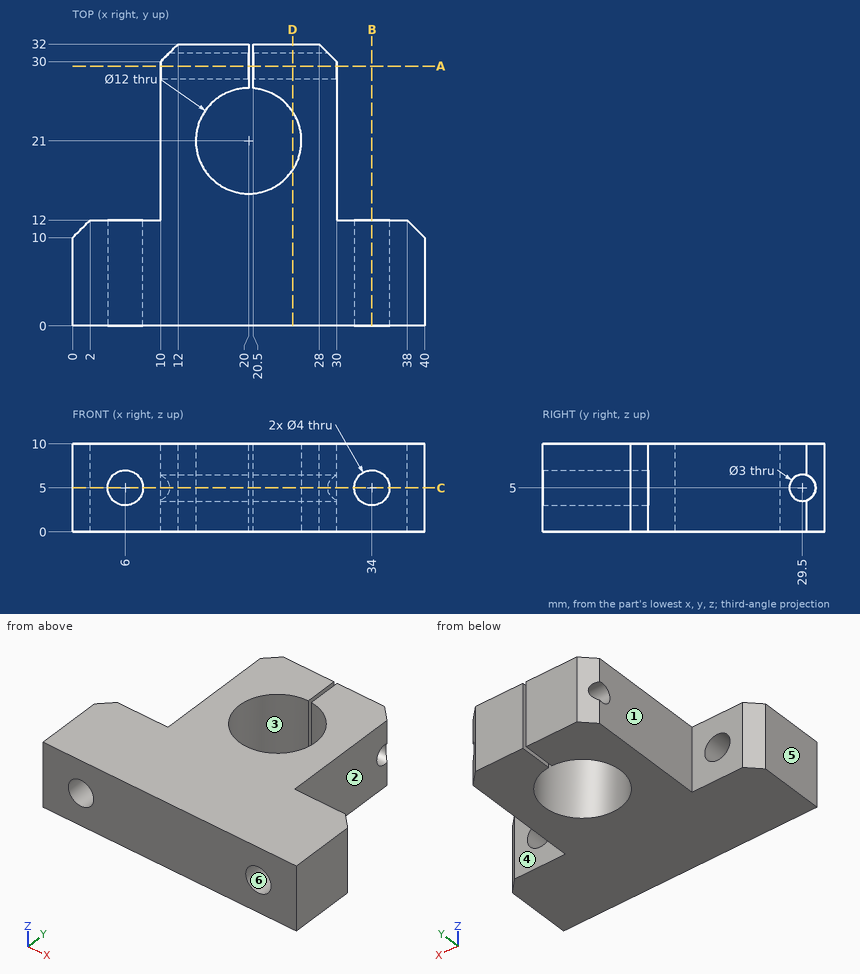
Geometry check sheet. Reference: drawing and pictorial views, mm from the part's lowest x, y, z. A direction names the side the tool comes from. Round coordinates to 2 decimals unless told otherwise and drop trailing zeros. Write each loop counter-clockwise with the first axis right and the second up, starting at its lowest first coordinate (ties: lowest second). Pieces come first, ordered by that corner, then holes. Notation, with made-up numbers: (-13.5, -11.75) -> (44.5, -11.75) arc R13 ccw to (44.5, 6.25) -> close; hole circle Ø3 at (1.5, 78). An arc over 180 degrees is marked (long way). Put each result on its own line as item: value.
1) Thickness scan on probe 1 along X at (y, z) = (11, 6.5); probe 2 along Y at (x, z) = (25, 4.5); probe 3 along Z at (x, y) = (34, 6.75). Record the ranges inside material, lowest first. Write a range as from..to.
Recorded:
probe 1: x = 1..4.68, 7.32..32.68, 35.32..39
probe 2: y = 0..17.68, 24.32..28.09, 30.91..32
probe 3: z = 0..3, 7..10
2) Cross-section at C-C, the plane z = 5. Give the number of separate pieces and of enclosed holes in the cut face, plus the area to 3 significant figures.
Recorded:
separate pieces: 5
enclosed holes: 0
area: 603 mm2
3) Access from +Z, -Z, +X, -X, +Y, -Y to the whole of each face (thin tool, end or side, straight path). Record for the marked faces 1, 2 and 3.
Recorded:
face 1: +Z, -Z, -X, +Y
face 2: +Z, -Z, +X, +Y
face 3: +Z, -Z
4) Cross-section at D-D, the plane x = 25. Enter the section's corners in (y, z).
Recorded:
outline: (0, 0) -> (17.68, 0) -> (17.68, 10) -> (0, 10) -> close; (24.32, 0) -> (32, 0) -> (32, 10) -> (24.32, 10) -> close; hole circle Ø3 at (29.5, 5)
5) Release check for a two-part mould opening along X. For the marked faces 4, 5 and 6 record: pulls with the +X half, pulls with the -X half, needs draft (parallel to the pull), parting line crosses it, or undercut.
Recorded:
face 4: needs draft
face 5: pulls with the -X half
face 6: undercut
6) Cross-section at A-A, the plane y = 29.5. Enter the section's corners in (x, z).
Recorded:
outline: (10, 0) -> (20, 0) -> (20, 3.5) -> (10, 3.5) -> close; (10, 6.5) -> (20, 6.5) -> (20, 10) -> (10, 10) -> close; (20.5, 0) -> (30, 0) -> (30, 3.5) -> (20.5, 3.5) -> close; (20.5, 6.5) -> (30, 6.5) -> (30, 10) -> (20.5, 10) -> close
7) Depth check by flat-ended pin: P1, Ø5, axis at y = 16.5, z = 6.5, coming from the +X side; P2, Ø1.5, axis at y = 30.5, z = 7, coming from the -X side; P3, Ø5, axis at x = 34.5, y = 26.5, coming from the +Z side; P4, Ø4, axis at x = 34, z = 4, coming from the +Y side. Enter the tip coordinate at first touch or a pass-through.
Recorded:
P1: stops at x = 30
P2: stops at x = 10
P3: passes through
P4: stops at y = 12
8) Cross-section at B-B, the plane x = 34. Enter the section's corners in (y, z), plus the area to 3 significant figures.
Recorded:
outline: (0, 0) -> (12, 0) -> (12, 3) -> (0, 3) -> close; (0, 7) -> (12, 7) -> (12, 10) -> (0, 10) -> close
area: 72.0 mm2
